from build123d import *

# Parameters (mm, degrees)
EXTRUDE_1_DEPTH     = 8
SKETCH_2_R          = 2
CUT_EXTRUDE_1_DEPTH = 5
FILLET_1_R          = 1


with BuildPart() as part:
    # 草图1 → 凸台-拉伸1 (new body)
    with BuildSketch(Plane(origin=(0, 0, 0), x_dir=(1, 0, 0), z_dir=(0, 1, 0))):
        with BuildLine():
            Line((-20, 0), (-2, 0))
            ThreePointArc((-2, 0), (-0.585786438, -0.585786438), (0, -2))
            Line((0, -2), (0, -15.720164609))
            Line((0, -15.720164609), (0, -21))
            Line((0, -21), (5, -21))
            Line((5, -21), (15, -21))
            Line((15, -21), (15, -16))
            Line((15, -16), (5, -16))
            Line((5, -16), (5, 0))
            Line((5, 0), (5, 5))
            Line((5, 5), (-20, 5))
            Line((-20, 5), (-20, 0))
        make_face()
    extrude(amount=EXTRUDE_1_DEPTH)

    # 草图2 → 切除-拉伸1 (cut)
    with BuildSketch(Plane(origin=(0, 0, 16), x_dir=(-1, 0, 0), z_dir=(0, 0, -1))):
        with Locations((-10, 4)):
            Circle(SKETCH_2_R)
    extrude(amount=-CUT_EXTRUDE_1_DEPTH, mode=Mode.SUBTRACT)

    # 圆角1
    fillet_1_edges = [part.edges().sort_by_distance(p)[0] for p in [
        (-20, 4, 0),
        (-20, 4, -5),
        (5, 4, -5),
        (15, 4, 16),
        (15, 4, 21),
        (0, 4, 21),
    ]]
    fillet(fillet_1_edges, radius=FILLET_1_R)


solid = part.part
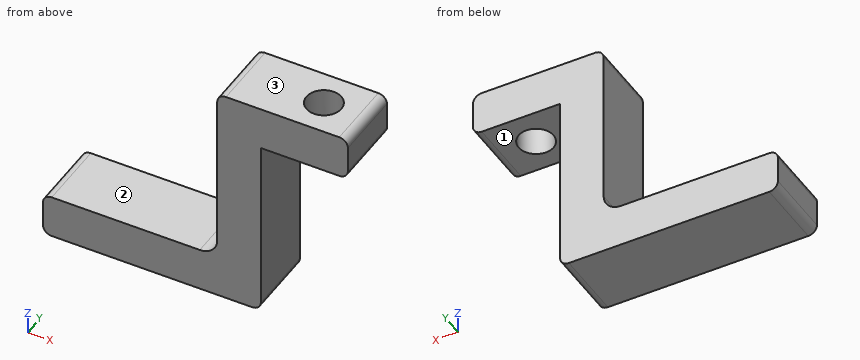
For this review, take the finished solid that the model builds, in its own axes (mm). Face numbers are marked on the shaded views. A direction names the side the tool comes from. Round coordinates to 2 decimals unless told otherwise and drop trailing zeros. Write each loop counter-clockwise with the first axis right and the second up, starting at its lowest first coordinate (ties: lowest second). Pieces come first, ordered by that corner, then holes. Notation, with made-up numbers: M -12,-8.75 L 2,-8.75 A37 ccw 2,29.25 Z; hole C 20,15.25 d4. An arc over 180 degrees is marked long. Write item = value, one per line. Start each with the question number.
(1) We need section A-A (y = 4). Give the boundary of the cut face in (x, z), then the cut area to 3 significant figures.
(2) We need section B-B (x = 10). Give the boundary of the cut face in (y, z).
(3) We need section D-D (z = -1.75). Give the boundary of the cut face in (x, y).
(4) We need section C-C (z = 18.75). Give the boundary of the cut face in (x, y).
(5) For the marked faces 1, 2 and 3, list the 3-axis set-ups (+Z, -Z, +X, -X, +Y, -Y) from which the entire face can be reached by the end or side of a thin tool; tool diameter is ignored.
(6) Clearance check with flat-ended pins moving along their axes: pin 1 Ø4.5 at (x, y) = (10, 4) entering from -Z; pin 2 Ø1.5 at (y, z) = (4.5, 17.5) entering from -X; pin 3 Ø4 at (y, z) = (5, 5) entering from +X. State where each tip first meets the part, or that it passes through.
(7) For line 1 along Y through (x, z) = (10, 17.6); line 2 along Z through (x, y) = (-14, 3.25); line 3 along Z through (x, y) = (12.5, 4.75), list the stretches that pass through material, from the lowest coordinate up.
Results found:
q1.outline = M -20,-4 A1 ccw -19,-5 L 4,-5 A1 ccw 5,-4 L 5,16 L 8,16 L 8,21 L 1,21 A1 ccw 0,20 L 0,2 A2 cw -2,0 L -19,0 A1 ccw -20,-1 Z; M 12,16 L 14,16 A1 ccw 15,17 L 15,20 A1 ccw 14,21 L 12,21 Z
q1.area = 260 mm²
q2.outline = M 0,16 L 2,16 L 2,21 L 0,21 Z; M 6,16 L 8,16 L 8,21 L 6,21 Z
q3.outline = M -20,0 L 5,0 L 5,8 L -20,8 Z
q4.outline = M 0,0 L 15,0 L 15,8 L 0,8 Z; hole C 10,4 d4
q5.face_1 = -Z, +X, +Y, -Y
q5.face_2 = +Z, -X, +Y, -Y
q5.face_3 = +Z, +X, -X, +Y, -Y
q6.pin_1 = 16
q6.pin_2 = 0
q6.pin_3 = 5
q7.line_1 = 0 to 2, 6 to 8
q7.line_2 = -5 to 0
q7.line_3 = 16 to 21
